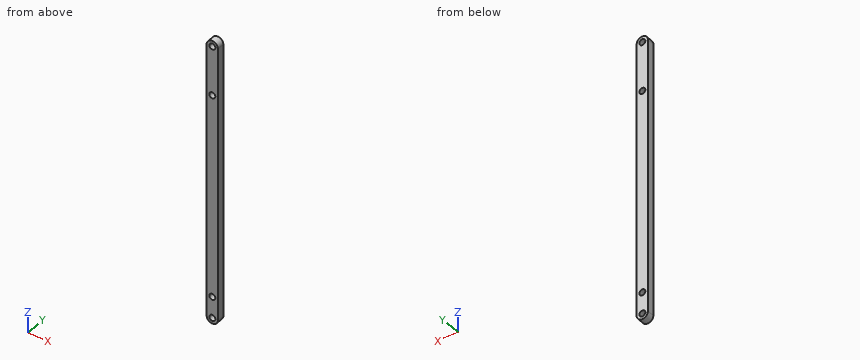
Autodesk Inventor part; units mm, degrees
ref_plane "YZ Plane" through (0, 0, 0) normal (1, 0, 0) x (0, 1, 0)
ref_plane "XZ Plane" through (0, 0, 0) normal (0, 1, 0) x (-1, 0, 0)
ref_plane "XY Plane" through (0, 0, 0) normal (0, 0, 1) x (1, 0, 0)
sketch "Sketch1" plane through (0, 0, 0) normal (0, 1, 0) x (-1, 0, 0)
  line L0 (0, 0) -> (0, -144.957) construction
  line L1 (3, 0) -> (3, -144.957)
  line L2 (-3, -144.957) -> (-3, 0)
  arc A0 (3, 0) -> (-3, 0) centre (0, 0) ccw
  arc A1 (-3, -144.957) -> (3, -144.957) centre (0, -144.957) ccw
  circle A2 centre (0, 0) radius 1.6
  circle A3 centre (0, -144.957) radius 1.6
  circle A4 centre (0, -26.085) radius 1.6
  circle A5 centre (0, -133.688) radius 1.6
  point P0 (0, -72.4785)
  dimension "d0" = 3.2
  dimension "d1" = 3.2
  dimension "d2" = 6
  dimension "d3" = 144.957
  dimension "d10" = 3.2
  dimension "d11" = 26.085
  dimension "d12" = 3.2
  dimension "d13" = 133.688
extrude "Extrusion1" add sketch "Sketch1" along normal blind 4
Could you check a few things on this model? Use its own coordinates, in mm. Round coordinates to 2 decimals unless told otherwise and drop trailing zeros. Order: outer loops, then holes, each group sorted by start corner. A loop starts at its lowest first (then second) coordinate and runs counter-clockwise, first axis right, second up. Notation, with made-up numbers: M -30,-8 L 7,-8 A11 ccw 7,13 Z; hole C -24.75,-29.75 d5. An arc over 180 degrees is marked long. One line per question, with ' | ' between items. Start each with the question number.
(1) For P1, Ø1.5, axis at x = 1, y = 3.5, coming from the +Z side, with a flat end and sliding along its axis, tell me the tip position at first contact or that it passes through.
(2) Suppose I cut it at B-B on y = 3.4. List the corners of the cut face in (x, z) for me (3 decimals).
(3) Suppose I cut it at A-A on x = 0. List the corners of the cut face in (y, z) for me (3 decimals), then the cut area to 3 significant figures.
(4) Please list where these lines run through material, in increasing order: line 1 along Z through (x, y) = (0, 1.4) (3 decimals); line 2 along Z through (x, y) = (-1.35, 2.25); line 3 along Z through (x, y) = (2.65, 2.05).
Geometry results:
1) P1: z = 2.99
2) outline: M -3,-144.957 A3 ccw 3,-144.957 L 3,0 A3 ccw -3,0 Z; hole C 0,-144.957 d3.2; hole C 0,-133.688 d3.2; hole C 0,-26.085 d3.2; hole C 0,0 d3.2
3) outline: M 0,-147.957 L 4,-147.957 L 4,-146.557 L 0,-146.557 Z; M 0,-143.357 L 4,-143.357 L 4,-135.288 L 0,-135.288 Z; M 0,-132.088 L 4,-132.088 L 4,-27.685 L 0,-27.685 Z; M 0,-24.485 L 4,-24.485 L 4,-1.6 L 0,-1.6 Z; M 0,1.6 L 4,1.6 L 4,3 L 0,3 Z | area: 553 mm²
4) line 1: -147.957 to -146.557, -143.357 to -135.288, -132.088 to -27.685, -24.485 to -1.6, 1.6 to 3 | line 2: -147.64 to -145.82, -144.1 to -134.55, -132.83 to -26.94, -25.23 to -0.86, 0.86 to 2.68 | line 3: -146.36 to 1.41
